For this review, use the dimensioned drawing (mm, ordinates from the lowest corner) and the shaded views. A direction names the side the tool comes from. Give positions to 0.01 mm unless a question says otherwise; leave off trailing zeros. Write each loop counter-clockwise with the first axis right and the second up, starting at its lowest first coordinate (ties: lowest second). Pieces come first, ordered by that corner, then holes.
1) Wall thickness on line 1 along Z through (x, y) = (8.25, 4.5); line 2 along X through (y, z) = (26, 43); line 3 along Y through (x, z) = (3.75, 7): over which ranges is each line inside the solid? List them lowest first.
2) Machinability: for the marked faces 1, 2 and 3, which of the approach directions +Z, -Z, +X, -X, +Y, -Y give a long, thin tool a straight path to every point of the face, cutting with its end or side? Answer none if there is none.
3) For P1, Ø2, axis at y = 26, z = 42, coming from the +X side; P2, Ø1.6, axis at x = 0.5, z = 35.5, coming from the -Y side; P3, Ø1, axis at y = 2, z = 58, coming from the -X side; P4, Ø12, axis at y = 8, z = 23, coming from the -X side (3 decimals), all flat-tipped, find the tip position at first contact; note any pin that passes through.
4) We need section A-A on y = 12. Give the boundary of the cut face in (x, z), and give its area (3 significant figures).
5) We need section B-B on z = 63. Give the boundary of the cut face in (x, y), and give its area (3 significant figures).
6) We need section C-C on x = 6.5. Give the boundary of the cut face in (y, z).
7) We need section D-D on y = 29. Give the boundary of the cut face in (x, z), and give its area (3 significant figures).
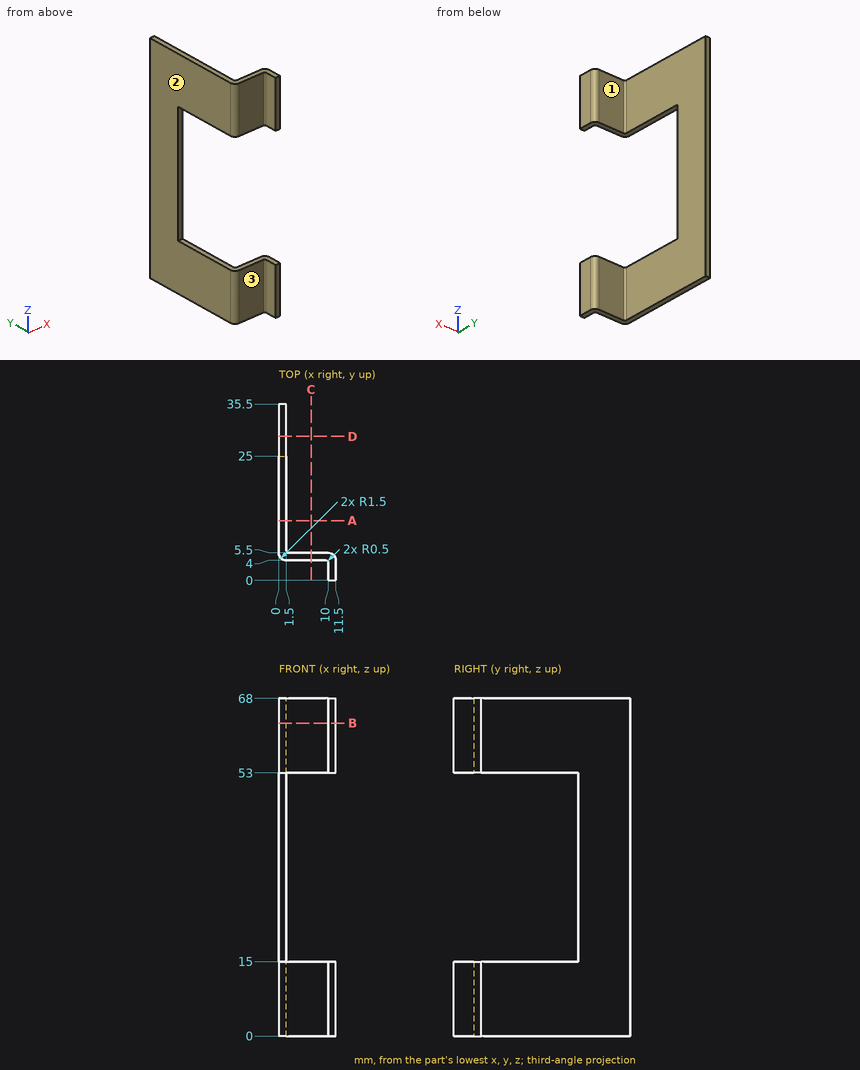
Results list:
1. line 1: z = 0 to 15, 53 to 68
1. line 2: x = 0 to 1.5
1. line 3: y = 4 to 5.5
2. face 1: +Z, -Z, +X, +Y
2. face 2: +Z, -Z, -X, +Y, -Y
2. face 3: +Z, -Z, -X, -Y
3. P1: stops at x = 1.5
3. P2: stops at y = 25
3. P3: stops at x = 10
3. P4: passes through
4. outline: (0, 0) - (1.5, 0) - (1.5, 15) - (0, 15) - close; (0, 53) - (1.5, 53) - (1.5, 68) - (0, 68) - close
4. area: 45.0 mm2
5. outline: (0, 5.5) arc R1.5 ccw to (1.5, 4) - (9.5, 4) arc R0.5 cw to (10, 3.5) - (10, 0) - (11.5, 0) - (11.5, 4) arc R1.5 ccw to (10, 5.5) - (2, 5.5) arc R0.5 cw to (1.5, 6) - (1.5, 35.5) - (0, 35.5) - close
5. area: 67.4 mm2
6. outline: (4, 0) - (5.5, 0) - (5.5, 15) - (4, 15) - close; (4, 53) - (5.5, 53) - (5.5, 68) - (4, 68) - close
7. outline: (0, 0) - (1.5, 0) - (1.5, 68) - (0, 68) - close
7. area: 102 mm2
